```python
from build123d import *

# Parameters (mm, degrees)
SKETCH1_W                          = 5.5
SKETCH1_H                          = 4
SKETCH2_R                          = 2.5
BOSS_EXTRUDE1_DEPTH                = 5
SKETCH3_R                          = 2.95
BOSS_EXTRUDE2_DEPTH                = 5.9
F_2_0_2_DIAMETER_HOLE1_D           = 2
F_2_0_2_DIAMETER_HOLE1_DEPTH       = 8
TAP_DRILL_FOR_M2_5X0_45_TAP1_D     = 2.05
TAP_DRILL_FOR_M2_5X0_45_TAP1_DEPTH = 6
TAP_DRILL_FOR_M2_5X0_45_TAP1_TIP   = 0.615882135
CHAMFER1_SIZE                      = 0.5
CHAMFER2_SIZE                      = 0.133974596
CHAMFER2_SIZE2                     = 0.5


with BuildPart() as part:
    # Sketch1 → Revolve1 (revolve)
    with BuildSketch(Plane.XY):
        with Locations((7.75, 2)):
            Rectangle(SKETCH1_W, SKETCH1_H)
    revolve(axis=Axis((5, 0, 0), (1, 0, 0)))

    # Sketch2 → Boss-Extrude1 (add)
    with BuildSketch(Plane.ZY.offset(-5)):
        Circle(SKETCH2_R)
    extrude(amount=BOSS_EXTRUDE1_DEPTH)

    # Sketch3 → Boss-Extrude2 (add)
    with BuildSketch(Plane(origin=(10.5, 0, 0), x_dir=(0, 0, -1), z_dir=(1, 0, 0))):
        Circle(SKETCH3_R)
    extrude(amount=BOSS_EXTRUDE2_DEPTH)

    # Ø2.0 (2) Diameter Hole1
    with Locations(Plane(origin=(8, -4, 0), x_dir=(0, 0, -1), z_dir=(0, -1, 0))):
        with Locations((0, 0)):
            Hole(F_2_0_2_DIAMETER_HOLE1_D / 2, depth=F_2_0_2_DIAMETER_HOLE1_DEPTH)

    # Tap Drill for M2.5x0.45 Tap1
    with Locations(Plane(origin=(16.4, 0, 0), x_dir=(0, 0, -1), z_dir=(1, 0, 0))):
        with Locations((0, 0)):
            Hole(TAP_DRILL_FOR_M2_5X0_45_TAP1_D / 2, depth=TAP_DRILL_FOR_M2_5X0_45_TAP1_DEPTH)
            with Locations((0, 0, -(TAP_DRILL_FOR_M2_5X0_45_TAP1_DEPTH + TAP_DRILL_FOR_M2_5X0_45_TAP1_TIP / 2))):  # 118° drill point
                Cone(0, TAP_DRILL_FOR_M2_5X0_45_TAP1_D / 2, TAP_DRILL_FOR_M2_5X0_45_TAP1_TIP, mode=Mode.SUBTRACT)

    # Chamfer1
    chamfer1_edges = [part.edges().sort_by_distance(p)[0] for p in [
        (0, 0, -2.5),
    ]]
    chamfer(chamfer1_edges, length=CHAMFER1_SIZE)

    # Chamfer2
    chamfer2_edges = [part.edges().sort_by_distance(p)[0] for p in [
        (5, -4, 0),
    ]]
    chamfer2_side = [part.faces().sort_by_distance(p)[0] for p in [
        (5, -3.886862915, 0),
    ]]
    chamfer(chamfer2_edges, length=CHAMFER2_SIZE, length2=CHAMFER2_SIZE2, reference=chamfer2_side[0])


solid = part.part
```
Source: CAD feature listing. Evaluate the final solid. Frame: model axes, mm. A direction names the side the tool comes from. Give positions to 0.01 mm unless a question says otherwise; leave off trailing zeros. Write each loop counter-clockwise with the first axis right and the second up, starting at its lowest first coordinate (ties: lowest second). Pieces come first, ordered by that corner, then holes. Notation, with made-up numbers: (12.5, 41) - (22.5, 41) arc R26 cw to (22.5, 75) - close; hole circle Ø9 at (79, 85.25). An arc over 180 degrees is marked (long way). One line per item, written item: value. Start each with the question number.
Q1. Set-up query: faces 1 (the face through (16.4, -1.3, 0)), 2 (the face through (13.358, 1.016, -0.133)), 3 (the face through (2.78, -2.44, -0.54)). Return all of +Z, -Z, +X, -X, +Y, -Y with unobstructed straight access to the full face (end or side cutting, diameter ignored); none if empty.
Q2. First-contact query: pin 1 Ø2 at (x, y) = (2.5, -0.5) entering from +Z; pin 2 Ø3 at (x, y) = (8, -3) entering from +Z. Flat tips, straight axial feed; report the tip coordinate or a pass-through.
Q3. Section query A-A, the plane x = 10.75. Return the cut outline in (y, z) (3 decimals).
Q4. Draft query along X for faces 4 (the face through (9, 0, 0)), 5 (the face through (5, 0, -3)), 6 (the face through (10.5, 2, -3)). Return one class per face: +X half, -X half, draft (parallel to the pull), parting line (faces both ways), or undercut.
Q5. Material intervals for probe 1 along Y at (x, z) = (13.2, 0) (3 decimals); probe 2 along Z at (x, y) = (8, 0.25); probe 3 along X at (y, z) = (-0.75, 0), sorted ascending. Write a range as from..to.
Q6. Section query B-B, the plane x = 8. Return the cut outline in (y, z).
Answer:
1. face 1: +Z, -Z, +X, +Y, -Y
1. face 2: +X
1. face 3: -X
2. pin 1: stops at z = 2.5
2. pin 2: stops at z = 3.71
3. outline: circle Ø5.9 at (0, 0); hole circle Ø2.05 at (0, 0)
4. face 4: undercut
4. face 5: -X half
4. face 6: +X half
5. probe 1: y = -2.95..-1.025, 1.025..2.95
5. probe 2: z = -3.99..-1, 1..3.99
5. probe 3: x = 0..7, 9..10.23
6. outline: (-3.87, -1) arc R4 ccw to (3.87, -1) - close; (-3.87, 1) - (3.87, 1) arc R4 ccw to start
